Work out the finished part from the listing and answer in its coordinate system (mm). Give positions to 0.01 mm unless a question says otherwise; leave off trailing zeros. Write each loop counter-clockwise with the first axis right and the second up, starting at its lowest first coordinate (ties: lowest second). Pieces come first, ordered by that corner, then holes. Notation, with made-up numbers: (53, 21.5) -> (60, 21.5) arc R20 cw to (60, 49.5) -> close; hole circle Ø10 at (57.25, 11.5). An arc over 180 degrees is marked (long way). Use a Markdown table: item, result. Add a question column.
Q1. Consider line 1 (X direction, y = 87.63, z = 3.75) (3 decimals); line 2 (Y direction, x = -8, z = 6); line 3 (X direction, y = 71.5, z = 2). Determine where each line is inside the solid, lowest interval first.
Q2. Section C-C, the plane x = 7 is taken. Give the vertices of the cut face in (y, z), plus the area to 3 significant figures.
Q3. Each of these flat-tipped pins is pushed along its axis until it touches: pin 1 Ø3 at (x, y) = (0, 95.25) entering from -Z; pin 2 Ø8 at (x, y) = (2.5, 102) entering from -Z. Where does it stop, or does it pass through?
Q4. Section A-A, the plane y = 80.01 is taken. Give the vertices of the cut face in (x, z) (3 decimals), plus the area to 3 significant figures.
Q5. Section B-B, the plane z = 2.75 is taken. State how many separate pieces and enclosed holes the cut face has, plus the area to 3 significant figures.
from build123d import *

# Parameters (mm, degrees)
SKETCH1_R           = 3.175
SKETCH1_R_2         = 1.905
SKETCH1_R_3         = 1.49987
BOSS_EXTRUDE1_DEPTH = 6.35


with BuildPart() as part:
    # Sketch1 → Boss-Extrude1 (new body)
    with BuildSketch(Plane.XY):
        with BuildLine():
            Line((-10.922, 0), (-10.922, 190.5))
            ThreePointArc((-10.922, 190.5), (0, 201.422), (10.922, 190.5))
            Line((10.922, 190.5), (10.922, 0))
            ThreePointArc((10.922, 0), (0, -10.922), (-10.922, 0))
        make_face()
        Circle(SKETCH1_R, mode=Mode.SUBTRACT)
        with Locations((0, 95.25)):
            Circle(SKETCH1_R_2, mode=Mode.SUBTRACT)
        with Locations((0, 87.63)):
            Circle(SKETCH1_R_2, mode=Mode.SUBTRACT)
        with Locations((0, 80.01)):
            Circle(SKETCH1_R_2, mode=Mode.SUBTRACT)
        with Locations((0, 72.39)):
            Circle(SKETCH1_R_2, mode=Mode.SUBTRACT)
        with Locations((0, 102.87)):
            Circle(SKETCH1_R_2, mode=Mode.SUBTRACT)
        with Locations((0, 170.789184136)):
            Circle(SKETCH1_R_3, mode=Mode.SUBTRACT)
        with Locations((0, 158.089184136)):
            Circle(SKETCH1_R_3, mode=Mode.SUBTRACT)
    extrude(amount=BOSS_EXTRUDE1_DEPTH)


solid = part.part
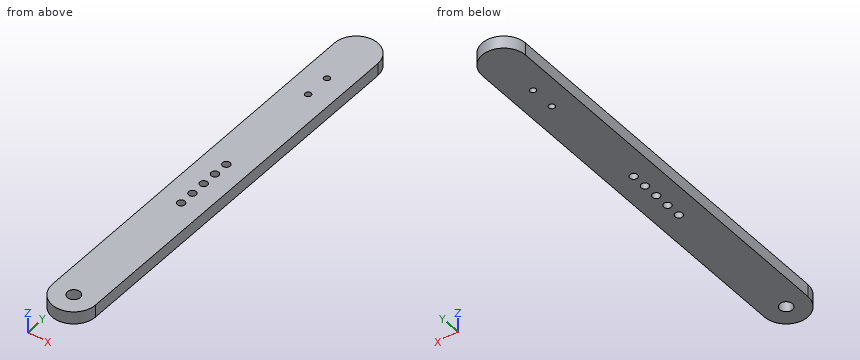
Result set:
| question | item | result |
|---|---|---|
| 1 | line 1 | x = -10.922 to -1.905, 1.905 to 10.922 |
| 1 | line 2 | y = -7.44 to 197.94 |
| 1 | line 3 | x = -10.92 to -1.68, 1.68 to 10.92 |
| 2 | outline | (-8.38, 0) -> (198.88, 0) -> (198.88, 6.35) -> (-8.38, 6.35) -> close |
| 2 | area | 1,320 mm2 |
| 3 | pin 1 | passes through |
| 3 | pin 2 | stops at z = 0 |
| 4 | outline | (-10.922, 0) -> (-1.905, 0) -> (-1.905, 6.35) -> (-10.922, 6.35) -> close; (1.905, 0) -> (10.922, 0) -> (10.922, 6.35) -> (1.905, 6.35) -> close |
| 4 | area | 115 mm2 |
| 5 | separate pieces | 1 |
| 5 | enclosed holes | 8 |
| 5 | area | 4,430 mm2 |
